Read the model definition and answer for the solid it produces. Units are mm, in the model's axes. Coordinates: 2 decimals unless noted, no trailing zeros. Loops run counter-clockwise (first coordinate to the right, second up) from the corner with the lowest first, then second, coordinate; pieces in that order, holes last. Notation, with made-up numbers: (19, -25.5) - (24, -25.5) arc R10 cw to (24, -13.5) - close; hole circle Ø1 at (-30, 3). An arc over 180 degrees is marked (long way). Use one line per item in the form item = value. Start each with the question number.
1) Each of these flat-tipped pins is pushed along its axis until it touches: P1, Ø7.5, axis at y = -44.21, z = 16.29, coming from the -X side; P2, Ø4, axis at x = 11, z = -81.5, coming from the +Y side; P3, Ø1, axis at x = 7, z = 79, coming from the +Y side; P4, Ø6, axis at x = 6, z = -17.5, coming from the +Y side. Where does it stop, or does it pass through?
2) A cutting plane is placed at D-D (y = 147.5). Give the vertices of the cut face in (x, z).
3) A cutting plane is placed at A-A (y = 33). Give the vertices of the cut face in (x, z).
4) The mould has two halves that part along Y. Classify faces 1 (the face through (9.658, -40.795, -79.955)), 2 (the face through (9, -229, -177.8)), 3 (the face through (9.39, -185.05, 32.53)): released by +Y, released by -Y, zero draft, split by the parting line, or undercut.
5) A cutting plane is placed at C-C (z = 155). Give the vertices of the cut face in (x, y).
6) A cutting plane is placed at B-B (x = 12). State how many separate pieces and enclosed holes the cut face has, and give its area (3 significant figures).
7) Consider line 1 (Y direction, x = 8.75, z = 19.5); line 2 (Z direction, x = 1.75, y = -42); line 3 (Y direction, x = 2.5, z = 12). Determine where each line is inside the solid, lowest interval first.
from build123d import *

# Parameters (mm, degrees)
F1_DEPTH = 19.05
F2_R     = 6.35
F3_DEPTH = 19.051


with BuildPart() as f1:
    # F0 (on Right) → F1 (new body)
    with BuildSketch(Plane.YZ):
        with BuildLine():
            ThreePointArc((-21.722689, 172.921289), (-186.770129, 29.95218), (-254, -177.8))
            Line((-254, -177.8), (-203.2, -177.8))
            ThreePointArc((-203.2, -177.8), (0, -152.4), (203.2, -177.8))
            Line((203.2, -177.8), (254, -177.8))
            ThreePointArc((254, -177.8), (251.689261, -148.097726), (247.208804, -118.64454))
            ThreePointArc((247.208804, -118.64454), (240.0276, -101.498698), (226.504407, -88.74437))
            ThreePointArc((226.504407, -88.74437), (116.258342, 9.959742), (48.659161, 141.591986))
            ThreePointArc((48.659161, 141.591986), (20.658526, 173.409755), (-21.722689, 172.921289))
        make_face()
    extrude(amount=F1_DEPTH)

    # F2 (on face) → F3 (cut, through all)
    with BuildSketch(Plane.YZ.offset(19.05)):
        with Locations((31.991019, -85.309384)):
            Circle(F2_R)
        with Locations((31.991019, -34.509384)):
            Circle(F2_R)
        with Locations((31.991019, 16.290616)):
            Circle(F2_R)
        with Locations((31.991019, 67.090616)):
            Circle(F2_R)
        with Locations((-44.208981, -85.309384)):
            Circle(F2_R)
        with Locations((-44.208981, -34.509384)):
            Circle(F2_R)
        with Locations((-44.208981, 16.290616)):
            Circle(F2_R)
        with Locations((-44.208981, 67.090616)):
            Circle(F2_R)
        with Locations((31.991019, 117.890616)):
            Circle(F2_R)
        with Locations((-44.208981, 117.890616)):
            Circle(F2_R)
    extrude(amount=-F3_DEPTH, mode=Mode.SUBTRACT)


solid = f1.part
Found:
q1.P1 = through
q1.P2 = 218.13
q1.P3 = 73.48
q1.P4 = 142.27
q2.outline = (0, -165.68) - (19.05, -165.68) - (19.05, -25.94) - (0, -25.94) - close
q3.outline = (0, -153.06) - (19.05, -153.06) - (19.05, -91.58) - (0, -91.58) - close; (0, -79.04) - (19.05, -79.04) - (19.05, -40.78) - (0, -40.78) - close; (0, -28.24) - (19.05, -28.24) - (19.05, 10.02) - (0, 10.02) - close; (0, 22.56) - (19.05, 22.56) - (19.05, 60.82) - (0, 60.82) - close; (0, 73.36) - (19.05, 73.36) - (19.05, 111.62) - (0, 111.62) - close; (0, 124.16) - (19.05, 124.16) - (19.05, 165.62) - (0, 165.62) - close
q4.face_1 = undercut
q4.face_2 = zero draft
q4.face_3 = released by -Y
q5.outline = (0, -55.42) - (19.05, -55.42) - (19.05, 42.39) - (0, 42.39) - close
q6.separate_pieces = 1
q6.enclosed_holes = 10
q6.area = 107,000 mm^2
q7.line_1 = -193.47 to -49.69, -38.73 to 26.51, 37.47 to 109.11
q7.line_2 = -153.47 to -91.26, -79.36 to -40.46, -28.56 to 10.34, 22.24 to 61.14, 73.04 to 111.94, 123.84 to 162.63
q7.line_3 = -198 to -48.89, -39.53 to 27.31, 36.67 to 114.69
